Check sheet for the modelled part. Datum: model origin and axes. Units: mm. Give positions to 0.01 mm unless a question says otherwise; leave off trailing zeros. Order: outer loops, then holes, each group sorted by start corner. A loop starts at its lowest first (then second) coordinate and runs counter-clockwise, first axis right, second up.
Item 1: Material ranges on line 1 along X through (y, z) = (150.5, -6); line 2 along Z through (x, y) = (1.5, 329), recorded low to high.
Item 2: Sectioned sample at B-B on z = -4.5. Count the separate pieces of the cut face and the enclosed holes in it, and give its area (3 significant figures).
Item 3: Sectioned sample at A-A on y = 310.5. Record the boundary of the cut face in (x, z).
Item 4: Gauge pin test, flat ends, axial feed: P1, Ø4, axis at x = 7.5, y = 205.66, coming from the +Z side; P2, Ø6, axis at x = 7, y = 71.5, coming from the -Z side; P3, Ø7, axis at y = 231.375, z = -4.5, coming from the -X side. Record the tip position at first contact, or that the pin passes through.
from build123d import *

# Parameters (mm, degrees)
BOSS_EXTRUDE1_DEPTH = 360
CUT_EXTRUDE1_REACH  = 2.5
SKETCH2_R           = 2.25
CUT_EXTRUDE2_REACH  = 14
SKETCH3_R           = 2.25


with BuildPart() as part:
    # Sketch1 → Boss-Extrude1 (new body)
    with BuildSketch(Plane(origin=(0, 0, 0), x_dir=(1, 0, 0), z_dir=(0, 1, 0))):
        Polygon((0, 0), (15, 0), (15, 12), (14.5, 12), (14.5, 0.5), (0, 0.5), align=None)
    extrude(amount=BOSS_EXTRUDE1_DEPTH)

    # Sketch2 → Cut-Extrude1 (cut, up to next)
    with BuildSketch(Plane.ZY.offset(-14.5), mode=Mode.PRIVATE) as cut_extrude1_sk1:
        with Locations((-4.5, 355.5)):
            Circle(SKETCH2_R)
    cut_extrude1_tool1 = extrude(cut_extrude1_sk1.sketch, amount=-CUT_EXTRUDE1_REACH, mode=Mode.PRIVATE) & part.part
    add(cut_extrude1_tool1.solids().sort_by_distance((14.5, 355.5, -4.5))[0], mode=Mode.SUBTRACT)
    # Sketch2 → Cut-Extrude1 (cut, up to next)
    with BuildSketch(Plane.ZY.offset(-14.5), mode=Mode.PRIVATE) as cut_extrude1_sk2:
        with Locations((-4.5, 329.8125)):
            Circle(SKETCH2_R)
    cut_extrude1_tool2 = extrude(cut_extrude1_sk2.sketch, amount=-CUT_EXTRUDE1_REACH, mode=Mode.PRIVATE) & part.part
    add(cut_extrude1_tool2.solids().sort_by_distance((14.5, 329.8125, -4.5))[0], mode=Mode.SUBTRACT)
    # Sketch2 → Cut-Extrude1 (cut, up to next)
    with BuildSketch(Plane.ZY.offset(-14.5), mode=Mode.PRIVATE) as cut_extrude1_sk3:
        with Locations((-4.5, 304.125)):
            Circle(SKETCH2_R)
    cut_extrude1_tool3 = extrude(cut_extrude1_sk3.sketch, amount=-CUT_EXTRUDE1_REACH, mode=Mode.PRIVATE) & part.part
    add(cut_extrude1_tool3.solids().sort_by_distance((14.5, 304.125, -4.5))[0], mode=Mode.SUBTRACT)
    # Sketch2 → Cut-Extrude1 (cut, up to next)
    with BuildSketch(Plane.ZY.offset(-14.5), mode=Mode.PRIVATE) as cut_extrude1_sk4:
        with Locations((-4.5, 278.4375)):
            Circle(SKETCH2_R)
    cut_extrude1_tool4 = extrude(cut_extrude1_sk4.sketch, amount=-CUT_EXTRUDE1_REACH, mode=Mode.PRIVATE) & part.part
    add(cut_extrude1_tool4.solids().sort_by_distance((14.5, 278.4375, -4.5))[0], mode=Mode.SUBTRACT)
    # Sketch2 → Cut-Extrude1 (cut, up to next)
    with BuildSketch(Plane.ZY.offset(-14.5), mode=Mode.PRIVATE) as cut_extrude1_sk5:
        with Locations((-4.5, 252.75)):
            Circle(SKETCH2_R)
    cut_extrude1_tool5 = extrude(cut_extrude1_sk5.sketch, amount=-CUT_EXTRUDE1_REACH, mode=Mode.PRIVATE) & part.part
    add(cut_extrude1_tool5.solids().sort_by_distance((14.5, 252.75, -4.5))[0], mode=Mode.SUBTRACT)
    # Sketch2 → Cut-Extrude1 (cut, up to next)
    with BuildSketch(Plane.ZY.offset(-14.5), mode=Mode.PRIVATE) as cut_extrude1_sk6:
        with Locations((-4.5, 231.375)):
            Circle(SKETCH2_R)
    cut_extrude1_tool6 = extrude(cut_extrude1_sk6.sketch, amount=-CUT_EXTRUDE1_REACH, mode=Mode.PRIVATE) & part.part
    add(cut_extrude1_tool6.solids().sort_by_distance((14.5, 231.375, -4.5))[0], mode=Mode.SUBTRACT)
    # Sketch2 → Cut-Extrude1 (cut, up to next)
    with BuildSketch(Plane.ZY.offset(-14.5), mode=Mode.PRIVATE) as cut_extrude1_sk7:
        with Locations((-4.5, 205.6875)):
            Circle(SKETCH2_R)
    cut_extrude1_tool7 = extrude(cut_extrude1_sk7.sketch, amount=-CUT_EXTRUDE1_REACH, mode=Mode.PRIVATE) & part.part
    add(cut_extrude1_tool7.solids().sort_by_distance((14.5, 205.6875, -4.5))[0], mode=Mode.SUBTRACT)
    # Sketch2 → Cut-Extrude1 (cut, up to next)
    with BuildSketch(Plane.ZY.offset(-14.5), mode=Mode.PRIVATE) as cut_extrude1_sk8:
        with Locations((-4.5, 180)):
            Circle(SKETCH2_R)
    cut_extrude1_tool8 = extrude(cut_extrude1_sk8.sketch, amount=-CUT_EXTRUDE1_REACH, mode=Mode.PRIVATE) & part.part
    add(cut_extrude1_tool8.solids().sort_by_distance((14.5, 180, -4.5))[0], mode=Mode.SUBTRACT)
    # Sketch2 → Cut-Extrude1 (cut, up to next)
    with BuildSketch(Plane.ZY.offset(-14.5), mode=Mode.PRIVATE) as cut_extrude1_sk9:
        with Locations((-4.5, 154.3125)):
            Circle(SKETCH2_R)
    cut_extrude1_tool9 = extrude(cut_extrude1_sk9.sketch, amount=-CUT_EXTRUDE1_REACH, mode=Mode.PRIVATE) & part.part
    add(cut_extrude1_tool9.solids().sort_by_distance((14.5, 154.3125, -4.5))[0], mode=Mode.SUBTRACT)
    # Sketch2 → Cut-Extrude1 (cut, up to next)
    with BuildSketch(Plane.ZY.offset(-14.5), mode=Mode.PRIVATE) as cut_extrude1_sk10:
        with Locations((-4.5, 128.625)):
            Circle(SKETCH2_R)
    cut_extrude1_tool10 = extrude(cut_extrude1_sk10.sketch, amount=-CUT_EXTRUDE1_REACH, mode=Mode.PRIVATE) & part.part
    add(cut_extrude1_tool10.solids().sort_by_distance((14.5, 128.625, -4.5))[0], mode=Mode.SUBTRACT)
    # Sketch2 → Cut-Extrude1 (cut, up to next)
    with BuildSketch(Plane.ZY.offset(-14.5), mode=Mode.PRIVATE) as cut_extrude1_sk11:
        with Locations((-4.5, 107.25)):
            Circle(SKETCH2_R)
    cut_extrude1_tool11 = extrude(cut_extrude1_sk11.sketch, amount=-CUT_EXTRUDE1_REACH, mode=Mode.PRIVATE) & part.part
    add(cut_extrude1_tool11.solids().sort_by_distance((14.5, 107.25, -4.5))[0], mode=Mode.SUBTRACT)
    # Sketch2 → Cut-Extrude1 (cut, up to next)
    with BuildSketch(Plane.ZY.offset(-14.5), mode=Mode.PRIVATE) as cut_extrude1_sk12:
        with Locations((-4.5, 81.5625)):
            Circle(SKETCH2_R)
    cut_extrude1_tool12 = extrude(cut_extrude1_sk12.sketch, amount=-CUT_EXTRUDE1_REACH, mode=Mode.PRIVATE) & part.part
    add(cut_extrude1_tool12.solids().sort_by_distance((14.5, 81.5625, -4.5))[0], mode=Mode.SUBTRACT)
    # Sketch2 → Cut-Extrude1 (cut, up to next)
    with BuildSketch(Plane.ZY.offset(-14.5), mode=Mode.PRIVATE) as cut_extrude1_sk13:
        with Locations((-4.5, 55.875)):
            Circle(SKETCH2_R)
    cut_extrude1_tool13 = extrude(cut_extrude1_sk13.sketch, amount=-CUT_EXTRUDE1_REACH, mode=Mode.PRIVATE) & part.part
    add(cut_extrude1_tool13.solids().sort_by_distance((14.5, 55.875, -4.5))[0], mode=Mode.SUBTRACT)
    # Sketch2 → Cut-Extrude1 (cut, up to next)
    with BuildSketch(Plane.ZY.offset(-14.5), mode=Mode.PRIVATE) as cut_extrude1_sk14:
        with Locations((-4.5, 30.1875)):
            Circle(SKETCH2_R)
    cut_extrude1_tool14 = extrude(cut_extrude1_sk14.sketch, amount=-CUT_EXTRUDE1_REACH, mode=Mode.PRIVATE) & part.part
    add(cut_extrude1_tool14.solids().sort_by_distance((14.5, 30.1875, -4.5))[0], mode=Mode.SUBTRACT)
    # Sketch2 → Cut-Extrude1 (cut, up to next)
    with BuildSketch(Plane.ZY.offset(-14.5), mode=Mode.PRIVATE) as cut_extrude1_sk15:
        with Locations((-4.5, 4.5)):
            Circle(SKETCH2_R)
    cut_extrude1_tool15 = extrude(cut_extrude1_sk15.sketch, amount=-CUT_EXTRUDE1_REACH, mode=Mode.PRIVATE) & part.part
    add(cut_extrude1_tool15.solids().sort_by_distance((14.5, 4.5, -4.5))[0], mode=Mode.SUBTRACT)

    # Sketch3 → Cut-Extrude2 (cut, up to next)
    with BuildSketch(Plane.XY, mode=Mode.PRIVATE) as cut_extrude2_sk1:
        with Locations((7.5, 355.5)):
            Circle(SKETCH3_R)
    cut_extrude2_tool1 = extrude(cut_extrude2_sk1.sketch, amount=-CUT_EXTRUDE2_REACH, mode=Mode.PRIVATE) & part.part
    add(cut_extrude2_tool1.solids().sort_by_distance((7.5, 355.5, 0))[0], mode=Mode.SUBTRACT)
    # Sketch3 → Cut-Extrude2 (cut, up to next)
    with BuildSketch(Plane.XY, mode=Mode.PRIVATE) as cut_extrude2_sk2:
        with Locations((7.5, 329.84375)):
            Circle(SKETCH3_R)
    cut_extrude2_tool2 = extrude(cut_extrude2_sk2.sketch, amount=-CUT_EXTRUDE2_REACH, mode=Mode.PRIVATE) & part.part
    add(cut_extrude2_tool2.solids().sort_by_distance((7.5, 329.84375, 0))[0], mode=Mode.SUBTRACT)
    # Sketch3 → Cut-Extrude2 (cut, up to next)
    with BuildSketch(Plane.XY, mode=Mode.PRIVATE) as cut_extrude2_sk3:
        with Locations((7.5, 304.1875)):
            Circle(SKETCH3_R)
    cut_extrude2_tool3 = extrude(cut_extrude2_sk3.sketch, amount=-CUT_EXTRUDE2_REACH, mode=Mode.PRIVATE) & part.part
    add(cut_extrude2_tool3.solids().sort_by_distance((7.5, 304.1875, 0))[0], mode=Mode.SUBTRACT)
    # Sketch3 → Cut-Extrude2 (cut, up to next)
    with BuildSketch(Plane.XY, mode=Mode.PRIVATE) as cut_extrude2_sk4:
        with Locations((7.5, 278.53125)):
            Circle(SKETCH3_R)
    cut_extrude2_tool4 = extrude(cut_extrude2_sk4.sketch, amount=-CUT_EXTRUDE2_REACH, mode=Mode.PRIVATE) & part.part
    add(cut_extrude2_tool4.solids().sort_by_distance((7.5, 278.53125, 0))[0], mode=Mode.SUBTRACT)
    # Sketch3 → Cut-Extrude2 (cut, up to next)
    with BuildSketch(Plane.XY, mode=Mode.PRIVATE) as cut_extrude2_sk5:
        with Locations((7.5, 252.875)):
            Circle(SKETCH3_R)
    cut_extrude2_tool5 = extrude(cut_extrude2_sk5.sketch, amount=-CUT_EXTRUDE2_REACH, mode=Mode.PRIVATE) & part.part
    add(cut_extrude2_tool5.solids().sort_by_distance((7.5, 252.875, 0))[0], mode=Mode.SUBTRACT)
    # Sketch3 → Cut-Extrude2 (cut, up to next)
    with BuildSketch(Plane.XY, mode=Mode.PRIVATE) as cut_extrude2_sk6:
        with Locations((7.5, 231.3125)):
            Circle(SKETCH3_R)
    cut_extrude2_tool6 = extrude(cut_extrude2_sk6.sketch, amount=-CUT_EXTRUDE2_REACH, mode=Mode.PRIVATE) & part.part
    add(cut_extrude2_tool6.solids().sort_by_distance((7.5, 231.3125, 0))[0], mode=Mode.SUBTRACT)
    # Sketch3 → Cut-Extrude2 (cut, up to next)
    with BuildSketch(Plane.XY, mode=Mode.PRIVATE) as cut_extrude2_sk7:
        with Locations((7.5, 205.65625)):
            Circle(SKETCH3_R)
    cut_extrude2_tool7 = extrude(cut_extrude2_sk7.sketch, amount=-CUT_EXTRUDE2_REACH, mode=Mode.PRIVATE) & part.part
    add(cut_extrude2_tool7.solids().sort_by_distance((7.5, 205.65625, 0))[0], mode=Mode.SUBTRACT)
    # Sketch3 → Cut-Extrude2 (cut, up to next)
    with BuildSketch(Plane.XY, mode=Mode.PRIVATE) as cut_extrude2_sk8:
        with Locations((7.5, 180)):
            Circle(SKETCH3_R)
    cut_extrude2_tool8 = extrude(cut_extrude2_sk8.sketch, amount=-CUT_EXTRUDE2_REACH, mode=Mode.PRIVATE) & part.part
    add(cut_extrude2_tool8.solids().sort_by_distance((7.5, 180, 0))[0], mode=Mode.SUBTRACT)
    # Sketch3 → Cut-Extrude2 (cut, up to next)
    with BuildSketch(Plane.XY, mode=Mode.PRIVATE) as cut_extrude2_sk9:
        with Locations((7.5, 154.34375)):
            Circle(SKETCH3_R)
    cut_extrude2_tool9 = extrude(cut_extrude2_sk9.sketch, amount=-CUT_EXTRUDE2_REACH, mode=Mode.PRIVATE) & part.part
    add(cut_extrude2_tool9.solids().sort_by_distance((7.5, 154.34375, 0))[0], mode=Mode.SUBTRACT)
    # Sketch3 → Cut-Extrude2 (cut, up to next)
    with BuildSketch(Plane.XY, mode=Mode.PRIVATE) as cut_extrude2_sk10:
        with Locations((7.5, 128.6875)):
            Circle(SKETCH3_R)
    cut_extrude2_tool10 = extrude(cut_extrude2_sk10.sketch, amount=-CUT_EXTRUDE2_REACH, mode=Mode.PRIVATE) & part.part
    add(cut_extrude2_tool10.solids().sort_by_distance((7.5, 128.6875, 0))[0], mode=Mode.SUBTRACT)
    # Sketch3 → Cut-Extrude2 (cut, up to next)
    with BuildSketch(Plane.XY, mode=Mode.PRIVATE) as cut_extrude2_sk11:
        with Locations((7.5, 107.125)):
            Circle(SKETCH3_R)
    cut_extrude2_tool11 = extrude(cut_extrude2_sk11.sketch, amount=-CUT_EXTRUDE2_REACH, mode=Mode.PRIVATE) & part.part
    add(cut_extrude2_tool11.solids().sort_by_distance((7.5, 107.125, 0))[0], mode=Mode.SUBTRACT)
    # Sketch3 → Cut-Extrude2 (cut, up to next)
    with BuildSketch(Plane.XY, mode=Mode.PRIVATE) as cut_extrude2_sk12:
        with Locations((7.5, 81.46875)):
            Circle(SKETCH3_R)
    cut_extrude2_tool12 = extrude(cut_extrude2_sk12.sketch, amount=-CUT_EXTRUDE2_REACH, mode=Mode.PRIVATE) & part.part
    add(cut_extrude2_tool12.solids().sort_by_distance((7.5, 81.46875, 0))[0], mode=Mode.SUBTRACT)
    # Sketch3 → Cut-Extrude2 (cut, up to next)
    with BuildSketch(Plane.XY, mode=Mode.PRIVATE) as cut_extrude2_sk13:
        with Locations((7.5, 55.8125)):
            Circle(SKETCH3_R)
    cut_extrude2_tool13 = extrude(cut_extrude2_sk13.sketch, amount=-CUT_EXTRUDE2_REACH, mode=Mode.PRIVATE) & part.part
    add(cut_extrude2_tool13.solids().sort_by_distance((7.5, 55.8125, 0))[0], mode=Mode.SUBTRACT)
    # Sketch3 → Cut-Extrude2 (cut, up to next)
    with BuildSketch(Plane.XY, mode=Mode.PRIVATE) as cut_extrude2_sk14:
        with Locations((7.5, 30.15625)):
            Circle(SKETCH3_R)
    cut_extrude2_tool14 = extrude(cut_extrude2_sk14.sketch, amount=-CUT_EXTRUDE2_REACH, mode=Mode.PRIVATE) & part.part
    add(cut_extrude2_tool14.solids().sort_by_distance((7.5, 30.15625, 0))[0], mode=Mode.SUBTRACT)
    # Sketch3 → Cut-Extrude2 (cut, up to next)
    with BuildSketch(Plane.XY, mode=Mode.PRIVATE) as cut_extrude2_sk15:
        with Locations((7.5, 4.5)):
            Circle(SKETCH3_R)
    cut_extrude2_tool15 = extrude(cut_extrude2_sk15.sketch, amount=-CUT_EXTRUDE2_REACH, mode=Mode.PRIVATE) & part.part
    add(cut_extrude2_tool15.solids().sort_by_distance((7.5, 4.5, 0))[0], mode=Mode.SUBTRACT)


solid = part.part
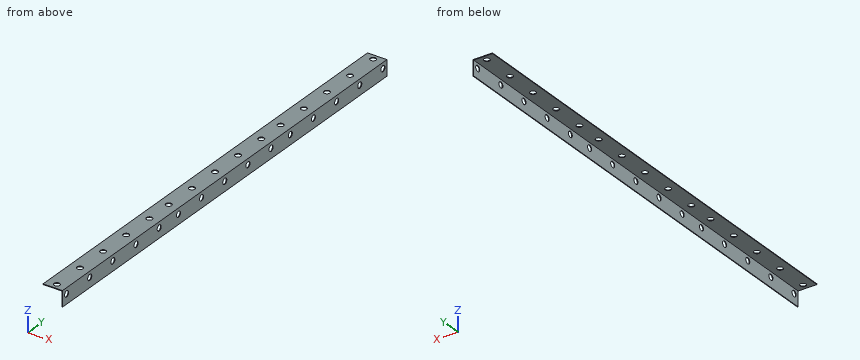
Report:
1. line 1: x = 14.5 to 15
1. line 2: z = -0.5 to 0
2. separate pieces: 16
2. enclosed holes: 0
2. area: 146 mm2
3. outline: (0, -0.5) - (14.5, -0.5) - (14.5, -12) - (15, -12) - (15, 0) - (0, 0) - close
4. P1: passes through
4. P2: stops at z = -0.5
4. P3: stops at x = 14.5
